Study the drawing (mm; zero at the part's minimum x, y, z) and answer. A direction names the side the tool comes from. Round coordinates to 2 decimals unless told otherwise and drop trailing zeros. Write each loop counter-clockwise with the first axis right and the second up, starting at its lowest first coordinate (ties: lowest second). Pieces come first, ordered by that corner, then holes. Notation, with made-up numbers: (13.5, 48.25) -> (17.5, 48.25) arc R16 cw to (17.5, 64.25) -> close; hole circle Ø5 at (44, 57). An arc over 180 degrees is marked (long way). Return JSON: item names as keys, results as strings.
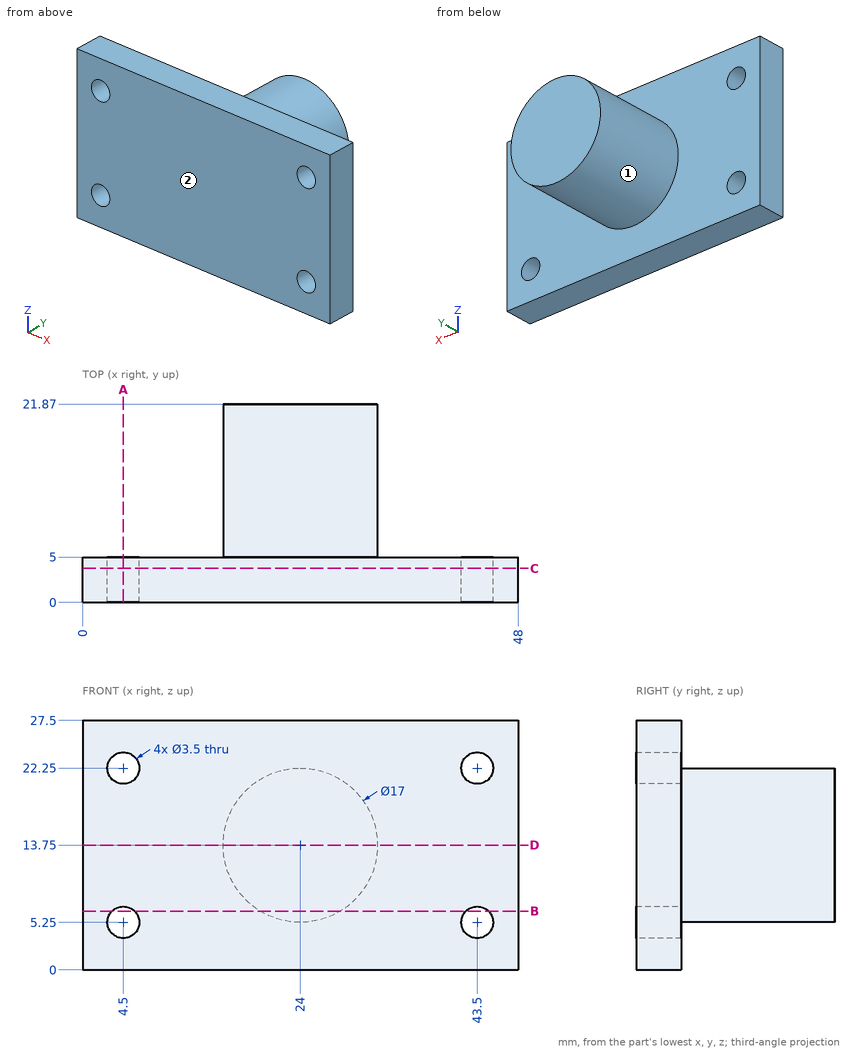
Item 1: Flat-ended cylindrical pins translate along their axes: pin 1 (10 mm diameter, centred on y = 16.5, z = 4.5, fed in from +X); pin 2 (8 mm diameter, centred on y = 16.5, z = 18.5, fed in from -X); pin 3 (4 mm diameter, centred on x = 4.5, z = 5.25, fed in from +Y). Find the tip coordinate at first contact, or state that the pin passes through.
Worked answers:
{"pin 1": "stops at x = 31.36", "pin 2": "stops at x = 15.53", "pin 3": "stops at y = 5"}
Item 2: Section B-B (z = 6.5) is taken. Give the vertices of the cut face in (x, y).
Worked answers:
{"outline": "(0, 0) -> (3.28, 0) -> (3.28, 5) -> (0, 5) -> close; (5.72, 0) -> (42.28, 0) -> (42.28, 5) -> (28.44, 5) -> (28.44, 21.87) -> (19.56, 21.87) -> (19.56, 5) -> (5.72, 5) -> close; (44.72, 0) -> (48, 0) -> (48, 5) -> (44.72, 5) -> close"}
Item 3: Straight lines are drawn through the part: L1, parallel to Z at x = 4.5, y = 2.8; L2, parallel to X at y = 2.3, z = 5.25; L3, parallel to Y at x = 13, z = 4. For each, find the intervals that lie inside material, in ascending order. Write a range as [from, to].
Worked answers:
{"L1": "z = [0, 3.5], [7, 20.5], [24, 27.5]", "L2": "x = [0, 2.75], [6.25, 41.75], [45.25, 48]", "L3": "y = [0, 5]"}
Item 4: Section A-A (x = 4.5) is taken. Give the vertices of the cut face in (y, z), then the cut area to 4 significant figures.
Worked answers:
{"outline": "(0, 0) -> (5, 0) -> (5, 3.5) -> (0, 3.5) -> close; (0, 7) -> (5, 7) -> (5, 20.5) -> (0, 20.5) -> close; (0, 24) -> (5, 24) -> (5, 27.5) -> (0, 27.5) -> close", "area": "102.5 mm2"}
Item 5: Section C-C (y = 3.75) is taken. Give the vertices of the cut face in (x, z).
Worked answers:
{"outline": "(0, 0) -> (48, 0) -> (48, 27.5) -> (0, 27.5) -> close; hole circle Ø3.5 at (4.5, 5.25); hole circle Ø3.5 at (4.5, 22.25); hole circle Ø3.5 at (43.5, 5.25); hole circle Ø3.5 at (43.5, 22.25)"}
Item 6: Section D-D (z = 13.75) is taken. Give the vertices of the cut face in (x, y).
Worked answers:
{"outline": "(0, 0) -> (48, 0) -> (48, 5) -> (32.5, 5) -> (32.5, 21.87) -> (15.5, 21.87) -> (15.5, 5) -> (0, 5) -> close"}
Item 7: A tool of negligible diameter and unlimited length cuts with its end or side. For the marked faces 1 and 2, from which of +Z, -Z, +X, -X, +Y, -Y can it reach the whole face along a straight path? Write none if from no direction.
Worked answers:
{"face 1": "+Y", "face 2": "+Z, -Z, +X, -X, -Y"}
